Build history of the part. All positions in model axes, mm. Face numbers are marked on the shaded views. A direction names the side the tool comes from. Give positions to 0.01 mm unless a question says otherwise; leave off trailing zeros. Order: outer loops, then holes, each group sorted by start corner. A loop starts at its lowest first (then second) coordinate and runs counter-clockwise, first axis right, second up. Notation, with made-up numbers: (-33.5, 30.25) - (11.5, 30.25) arc R25 cw to (11.5, 66.25) - close; hole circle Ø5 at (-30, 69). An arc over 180 degrees is marked (long way). One line per item, written item: value.
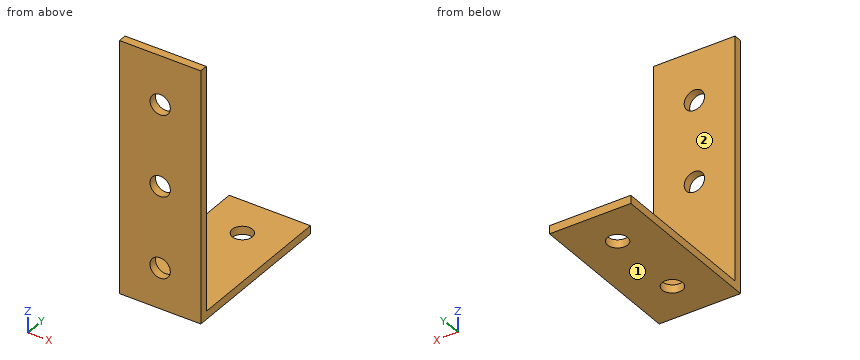
Autodesk Inventor part; units mm, degrees
ref_plane "YZ Plane" through (0, 0, 0) normal (1, 0, 0) x (0, 1, 0)
ref_plane "XZ Plane" through (0, 0, 0) normal (0, 1, 0) x (-1, 0, 0)
ref_plane "XY Plane" through (0, 0, 0) normal (0, 0, 1) x (1, 0, 0)
sketch "Sketch1" plane through (0, 0, 0) normal (0, 0, 1) x (1, 0, 0)
  line L0 (0, 0) -> (0, 50.8)
  line L1 (0, 50.8) -> (-25.4, 50.8)
  line L2 (-25.4, 50.8) -> (-25.4, 0)
  line L3 (-25.4, 0) -> (0, 0)
  dimension "d0" = 50.8
  dimension "d2" = 25.4
extrude "Extrusion1" add sketch "Sketch1" along normal blind 2.54
sketch "Sketch2" plane through (0, 0, 2.54) normal (0, 0, 1) x (1, 0, 0)
  line L0 (-25.4, 0) -> (-25.4, 2.54)
  line L1 (-25.4, 50.8) -> (-25.4, 0)
  line L2 (-25.4, 2.54) -> (0, 2.54)
  line L3 (0, 0) -> (0, 50.8)
  line L4 (0, 0) -> (-25.4, 0)
  line L5 (-25.4, 0) -> (0, 0)
  dimension "d5" = 2.54
extrude "Extrusion2" add sketch "Sketch2" along normal blind 76.2
hole "Hole1" at (-12.7, 2.54, 12.7) direction (0, -1, 0) diameter 6.35 end through all
pattern_linear "Rectangular Pattern1" count 3 spacing 25.4 along (0, 0, 1) of "Hole1"
hole "Hole2" at (-12.7, 12.7, 2.54) direction (0, 0, -1) diameter 6.35 end through all
pattern_linear "Rectangular Pattern2" count 2 spacing 25.4 along (0, 1, 0) of "Hole2"
properties part number "L-Gusset"
(1) Slice it at A-A, the plane z = 63.5. Give the cut face in (x, y) (3 decimals).
Completed:
outline: (-25.4, 0) - (-15.875, 0) - (-15.875, 2.54) - (-25.4, 2.54) - close; (-9.525, 0) - (0, 0) - (0, 2.54) - (-9.525, 2.54) - close
(2) Pin check, flat tip, straight feed: P1, Ø8, axis at x = -13.5, z = 42, coming from the +Y side. Stop position of the tip, or through.
Completed:
P1: y = 2.54
(3) Drill centre lines: line 1 (Z direction, x = -12.7, y = 2) (3 decimals); line 2 (Y direction, x = -12.7, z = 0.8) (3 decimals); line 3 (X direction, y = 1, z = 12.7) (3 decimals). Where is each one in solid material? Low to high.
Completed:
line 1: 0 to 9.525, 15.875 to 34.925, 41.275 to 60.325, 66.675 to 78.74
line 2: 0 to 9.525, 15.875 to 34.925, 41.275 to 50.8
line 3: -25.4 to -15.875, -9.525 to 0
(4) 3-axis set-ups, long thin cutter, end or side, ignore diameter. For the marked faces 1 and 2: which of +Z, -Z, +X, -X, +Y, -Y reach the whole face in a straight line?
Completed:
face 1: -Z, +X, -X, +Y, -Y
face 2: +Z, +X, -X, +Y
(5) Slice it at D-D, the plane y = 47.5. Give the cut face in (x, z), and give its area (3 significant figures).
Completed:
outline: (-25.4, 0) - (0, 0) - (0, 2.54) - (-25.4, 2.54) - close
area: 64.5 mm²
(6) Slice it at C-C, the plane x = -14.75. Give the cut face in (y, z), and give its area (3 significant figures).
Completed:
outline: (0, 0) - (10.28, 0) - (10.28, 2.54) - (2.54, 2.54) - (2.54, 10.28) - (0, 10.28) - close; (0, 15.12) - (2.54, 15.12) - (2.54, 35.68) - (0, 35.68) - close; (0, 40.52) - (2.54, 40.52) - (2.54, 61.08) - (0, 61.08) - close; (0, 65.92) - (2.54, 65.92) - (2.54, 78.74) - (0, 78.74) - close; (15.12, 0) - (35.68, 0) - (35.68, 2.54) - (15.12, 2.54) - close; (40.52, 0) - (50.8, 0) - (50.8, 2.54) - (40.52, 2.54) - close
area: 261 mm²
